Input: part model. Units: mm. Frame: model coordinates. A direction names the side the tool comes from. Coordinates: 2 decimals unless noted, no trailing zeros. Order: outer loops, then holes, each group sorted by start corner. A loop starts at its lowest first (then second) coordinate and runs counter-clockwise, first axis right, second up. Notation, with made-up numbers: (55, -31.5) -> (91, -31.5) arc R13 cw to (91, -21.5) -> close; hole circle Ø2 at (87, 46). An arc over 180 degrees is marked (long way). Use one line per item in the form item = value. Start each with the question number.
1) Section query B-B on x = 0. Output: boundary loops of the cut face in (y, z).
2) Ray query, line 1 along X through (y, z) = (0, 2.55); line 2 along Z through (x, y) = (7, 3); line 3 along X through (y, z) = (-7.5, 2.25). Return the intervals inside material, ascending.
3) Draft query along X for faces 5 (the flat face through (13.415, -7.764, 16.413)), 6 (the flat face through (8, 9, 18)). Return one class per face: pulls with the +X half, pulls with the -X half, needs draft (parallel to the pull), parting line crosses it, or undercut.
4) Section query A-A on z = 6. Count the separate pieces of the cut face and the enclosed holes in it, then the cut area to 3 significant figures.
5) Access query for faces 1 (the flat face through (0, 2, 0)), 2 (the flat face through (1.724, 12.486, 16.413)), 3 (the flat face through (-8.12, -10, 11)), 4 (the cylindrical face through (-0.17, 14.79, 9.34)). Directions: +Z, -Z, +X, -X, +Y, -Y. A direction counts if a zero-diameter tool reaches every point of the face in a straight line with its end or side. Return the directions, or none.
6) Pin query (flat end, axial travel): pin 1 (10 mm diameter, centred on x = 13, z = 3.5, fed in from +Y); pin 2 (13 mm diameter, centred on x = 0, y = 0, fed in from +Z); pin 3 (3 mm diameter, centred on y = -4, z = 7, fed in from -X); pin 4 (4.5 mm diameter, centred on x = 0, y = 13.5, fed in from -Z). Return the tip coordinate at first contact, or that it passes through.
7) Section query D-D on x = 6.5. Output: boundary loops of the cut face in (y, z).
8) Section query C-C on y = 0. Output: boundary loops of the cut face in (x, z), then the cut area to 3 significant figures.
from build123d import *

# Parameters (mm, degrees)
SKETCH2_R           = 17.4625
BOSS_EXTRUDE1_DEPTH = 18
SKETCH13_R          = 1.3
CUT_EXTRUDE6_DEPTH  = 15
SKETCH16_R          = 11
CUT_EXTRUDE9_DEPTH  = 15
CUT_EXTRUDE11_DEPTH = 22
SKETCH21_W          = 16.25
SKETCH21_H          = 2.78436417
CUT_EXTRUDE12_DEPTH = 31.559414466
CUT_EXTRUDE13_REACH = 32.559
SKETCH24_W          = 16.25
SKETCH24_H          = 6.70136321
CUT_EXTRUDE14_DEPTH = 17
SKETCH27_W          = 18.82071266
SKETCH27_H          = 0.75
CUT_EXTRUDE15_DEPTH = 31.559414466
CUT_EXTRUDE16_START = 14.3
CUT_EXTRUDE16_DEPTH = 1.8
SKETCH29_R          = 11
CUT_EXTRUDE17_DEPTH = 1.75


with BuildPart() as part:
    # Sketch2 → Boss-Extrude1 (new body)
    with BuildSketch(Plane.XY):
        Circle(SKETCH2_R)
    extrude(amount=BOSS_EXTRUDE1_DEPTH)

    # Sketch13 → Cut-Extrude6 (cut)
    with BuildSketch(Plane.XY.offset(18)):
        with Locations((0, 13.5)):
            Circle(SKETCH13_R)
        with Locations((11.691342951, -6.75)):
            Circle(SKETCH13_R)
        with Locations((-11.691342951, -6.75)):
            Circle(SKETCH13_R)
    extrude(amount=-CUT_EXTRUDE6_DEPTH, mode=Mode.SUBTRACT)

    # Sketch16 → Cut-Extrude9 (cut)
    with BuildSketch(Plane.XY.offset(18)):
        Circle(SKETCH16_R)
    extrude(amount=-CUT_EXTRUDE9_DEPTH, mode=Mode.SUBTRACT)

    # Sketch20 → Cut-Extrude11 (cut)
    with BuildSketch(Plane(origin=(5.95728493, 0, -11.08430825), x_dir=(0, 0, 1), z_dir=(0, 1, 0))):
        Polygon((16.52930825, -11.021800725), (16.52930825, -6.906800725), (14.92930825, -6.906800725), (14.92930825, -4.926800725), (16.52930825, -4.926800725), (16.52930825, -0.811800725), (18.05430825, -0.811800725), (18.05430825, 1.028199275), (22.11430825, 1.028199275), (22.11430825, -0.811800725), (23.63930825, -0.811800725), (23.63930825, -11.021800725), (22.11430825, -11.021800725), (22.11430825, -12.861800725), (18.05430825, -12.861800725), (18.05430825, -11.021800725), align=None)
    extrude(amount=-CUT_EXTRUDE11_DEPTH, mode=Mode.SUBTRACT)

    # Sketch21 → Cut-Extrude12 (cut, through all)
    with BuildSketch(Plane.XY.offset(18)):
        with Locations((0, -16.852182085)):
            Rectangle(SKETCH21_W, SKETCH21_H)
    extrude(amount=-CUT_EXTRUDE12_DEPTH, mode=Mode.SUBTRACT)

    # Cut-Extrude13: up to this face of the body (flat: up to its plane)
    cut_extrude13_end = Plane(part.part.faces().sort_by_distance((0, 0, 3))[0])
    # Sketch24 → Cut-Extrude13 (cut, up to the picked face)
    with BuildSketch(Plane.XY.offset(18), mode=Mode.PRIVATE) as cut_extrude13_sk1:
        with Locations((0.005436819, -10.109318395)):
            Rectangle(SKETCH24_W, SKETCH24_H)
    cut_extrude13_tool1 = split(extrude(cut_extrude13_sk1.sketch, amount=-CUT_EXTRUDE13_REACH, mode=Mode.PRIVATE), bisect_by=cut_extrude13_end, keep=Keep.BOTH, mode=Mode.PRIVATE)
    add(cut_extrude13_tool1.solids().sort_by(Axis((0.005437, -10.109318, 18), (0, 0, -1)))[0], mode=Mode.SUBTRACT)

    # Sketch26 → Cut-Extrude14 (cut)
    with BuildSketch(Plane.XY.offset(18)):
        Polygon((-8.119563181, -13.71), (-8.119563181, -15.46), (8.119563181, -15.46), (8.119563181, -13.71), (8.930436819, -13.71), (8.930436819, -12.71), (-8.919563181, -12.71), (-8.919563181, -13.71), align=None)
    extrude(amount=-CUT_EXTRUDE14_DEPTH, mode=Mode.SUBTRACT)

    # Sketch27 → Cut-Extrude15 (cut, through all)
    with BuildSketch(Plane.XY.offset(18)):
        with Locations((0, -15.085)):
            Rectangle(SKETCH27_W, SKETCH27_H)
    extrude(amount=-CUT_EXTRUDE15_DEPTH, mode=Mode.SUBTRACT)

    # Sketch28 → Cut-Extrude16 (cut)
    with BuildSketch(Plane.XY.offset(3).offset(CUT_EXTRUDE16_START)):
        Polygon((2.309401077, 13.5), (1.154700538, 15.5), (-1.154700538, 15.5), (-2.309401077, 13.5), (-1.154700538, 11.5), (1.154700538, 11.5), align=None)
        Polygon((-9.381941874, -6.75), (-10.536642413, -4.75), (-12.846043489, -4.75), (-14.000744028, -6.75), (-12.846043489, -8.75), (-10.536642413, -8.75), align=None)
        Polygon((14.000744028, -6.75), (12.846043489, -4.75), (10.536642413, -4.75), (9.381941874, -6.75), (10.536642413, -8.75), (12.846043489, -8.75), align=None)
    extrude(amount=-CUT_EXTRUDE16_DEPTH, mode=Mode.SUBTRACT)

    # Sketch29 → Cut-Extrude17 (cut)
    with BuildSketch(Plane.XY.offset(3)):
        Circle(SKETCH29_R)
    extrude(amount=-CUT_EXTRUDE17_DEPTH, mode=Mode.SUBTRACT)


solid = part.part
Answers below:
q1.outline = (-14.71, 0) -> (17.46, 0) -> (17.46, 18) -> (14.8, 18) -> (14.8, 17.3) -> (15.5, 17.3) -> (15.5, 15.5) -> (14.8, 15.5) -> (14.8, 3) -> (12.2, 3) -> (12.2, 15.5) -> (11.5, 15.5) -> (11.5, 17.3) -> (12.2, 17.3) -> (12.2, 18) -> (11, 18) -> (11, 1.25) -> (-11, 1.25) -> (-11, 3) -> (-12.71, 3) -> (-12.71, 1) -> (-14.71, 1) -> close
q2.line_1 = -17.46 to -11, 11 to 17.46
q2.line_2 = 0 to 1.25
q2.line_3 = -15.77 to -8.05, 8.05 to 15.77
q3.face_5 = undercut
q3.face_6 = needs draft
q4.separate_pieces = 1
q4.enclosed_holes = 3
q4.area = 447 mm^2
q5.face_1 = -Z, +X, -X, +Y, -Y
q5.face_2 = none
q5.face_3 = +Z, -Y
q5.face_4 = +Z
q6.pin_1 = 15.52
q6.pin_2 = 1.25
q6.pin_3 = -17.28
q6.pin_4 = 0
q7.outline = (-14.71, 0) -> (16.21, 0) -> (16.21, 18) -> (8.87, 18) -> (8.87, 1.25) -> (-8.87, 1.25) -> (-8.87, 3) -> (-12.71, 3) -> (-12.71, 1) -> (-14.71, 1) -> close
q8.outline = (-17.46, 0) -> (17.46, 0) -> (17.46, 18) -> (11, 18) -> (11, 1.25) -> (-11, 1.25) -> (-11, 18) -> (-17.46, 18) -> close
q8.area = 260 mm^2
